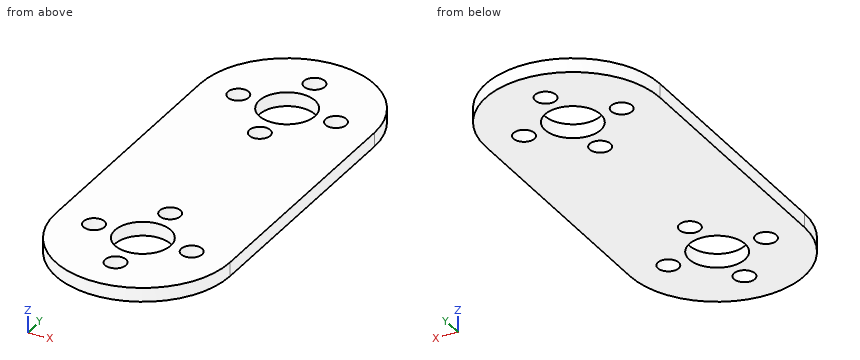
```python
from build123d import *

# Parameters (mm, degrees)
BOSS_EXTRUDE1_DEPTH     = 1
CUT_EXTRUDE1_REACH      = 53.093
SKETCH2_R               = 4
CUT_EXTRUDE2_REACH      = 53.093
SKETCH2_3_R             = 1.5
CIRPATTERN1_COUNT       = 4
MIRROR1_COPY_1_REACH    = 53.093
MIRROR1_COPY_1_SKETCH_R = 1.5
MIRROR1_COPY_2_REACH    = 53.093
MIRROR1_COPY_2_SKETCH_R = 1.5
MIRROR1_COPY_3_REACH    = 53.093
MIRROR1_COPY_3_SKETCH_R = 1.5


with BuildPart() as part:
    # Sketch1 → Boss-Extrude1 (new, symmetric)
    with BuildSketch(Plane.XY):
        with BuildLine():
            Line((-12.5, 0), (-12.5, 37))
            ThreePointArc((-12.5, 37), (0, 49.5), (12.5, 37))
            Line((12.5, 37), (12.5, 0))
            ThreePointArc((12.5, 0), (0, -12.5), (-12.5, 0))
        make_face()
    extrude(amount=BOSS_EXTRUDE1_DEPTH, both=True)

    # Sketch2 → Cut-Extrude1 (cut, up to next)
    with BuildSketch(Plane(origin=(0, 0, -1), x_dir=(-1, 0, 0), z_dir=(0, 0, -1)), mode=Mode.PRIVATE) as cut_extrude1_sk1:
        with Locations((0, 37)):
            Circle(SKETCH2_R)
    cut_extrude1_tool1 = extrude(cut_extrude1_sk1.sketch, amount=-CUT_EXTRUDE1_REACH, mode=Mode.PRIVATE) & part.part
    cut_extrude1 = cut_extrude1_tool1.solids().sort_by_distance((0, 37, -1))[0]
    add(cut_extrude1, mode=Mode.SUBTRACT)

    # Sketch2_3 → Cut-Extrude2 (cut, up to next)
    with BuildSketch(Plane(origin=(0, 0, -1), x_dir=(-1, 0, 0), z_dir=(0, 0, -1)), mode=Mode.PRIVATE) as cut_extrude2_sk1:
        with Locations((0, 44)):
            Circle(SKETCH2_3_R)
    cut_extrude2_tool1 = extrude(cut_extrude2_sk1.sketch, amount=-CUT_EXTRUDE2_REACH, mode=Mode.PRIVATE) & part.part
    cut_extrude2 = cut_extrude2_tool1.solids().sort_by_distance((0, 44, -1))[0]
    add(cut_extrude2, mode=Mode.SUBTRACT)

    # CirPattern1: Cut-Extrude2 ×4 about axis
    cirpattern1_axis = Axis((0, 37, 0), (0, 0, 1))
    for i in range(1, CIRPATTERN1_COUNT):
        add(cut_extrude2.rotate(cirpattern1_axis, i * 360 / CIRPATTERN1_COUNT), mode=Mode.SUBTRACT)

    # Mirror1: Cut-Extrude1, Cut-Extrude2 across plane
    add(cut_extrude1.mirror(Plane.ZX.offset(18.5)), mode=Mode.SUBTRACT)
    add(cut_extrude2.mirror(Plane.ZX.offset(18.5)), mode=Mode.SUBTRACT)

    # Mirror1 copy 1 sketch → Mirror1 copy 1 (cut, up to next)
    with BuildSketch(Plane(origin=(37, 0, -1), x_dir=(0, 1, 0), z_dir=(0, 0, -1)), mode=Mode.PRIVATE) as mirror1_copy_1_sk1:
        with Locations((0, -44)):
            Circle(MIRROR1_COPY_1_SKETCH_R)
    mirror1_copy_1_tool1 = extrude(mirror1_copy_1_sk1.sketch, amount=-MIRROR1_COPY_1_REACH, mode=Mode.PRIVATE) & part.part
    add(mirror1_copy_1_tool1.solids().sort_by_distance((-7, 0, -1))[0], mode=Mode.SUBTRACT)

    # Mirror1 copy 2 sketch → Mirror1 copy 2 (cut, up to next)
    with BuildSketch(Plane(origin=(0, -37, -1), x_dir=(1, 0, 0), z_dir=(0, 0, -1)), mode=Mode.PRIVATE) as mirror1_copy_2_sk1:
        with Locations((0, -44)):
            Circle(MIRROR1_COPY_2_SKETCH_R)
    mirror1_copy_2_tool1 = extrude(mirror1_copy_2_sk1.sketch, amount=-MIRROR1_COPY_2_REACH, mode=Mode.PRIVATE) & part.part
    add(mirror1_copy_2_tool1.solids().sort_by_distance((0, 7, -1))[0], mode=Mode.SUBTRACT)

    # Mirror1 copy 3 sketch → Mirror1 copy 3 (cut, up to next)
    with BuildSketch(Plane(origin=(-37, 0, -1), x_dir=(0, -1, 0), z_dir=(0, 0, -1)), mode=Mode.PRIVATE) as mirror1_copy_3_sk1:
        with Locations((0, -44)):
            Circle(MIRROR1_COPY_3_SKETCH_R)
    mirror1_copy_3_tool1 = extrude(mirror1_copy_3_sk1.sketch, amount=-MIRROR1_COPY_3_REACH, mode=Mode.PRIVATE) & part.part
    add(mirror1_copy_3_tool1.solids().sort_by_distance((7, 0, -1))[0], mode=Mode.SUBTRACT)


solid = part.part
```
Input: part model. Units: mm. Frame: model coordinates. Give positions to 0.01 mm unless a question says otherwise; leave off trailing zeros. Order: outer loops, then holes, each group sorted by start corner. A loop starts at its lowest first (then second) coordinate and runs counter-clockwise, first axis right, second up.
1. Cut plane D-D (y = -7). Return loops of the section in (x, z).
Computed:
outline: (-10.36, -1) - (-1.5, -1) - (-1.5, 1) - (-10.36, 1) - close; (1.5, -1) - (10.36, -1) - (10.36, 1) - (1.5, 1) - close
2. Pin query (flat end, axial travel): pin 1 Ø5 at (x, y) = (-7, 37) entering from +Z; pin 2 Ø1 at (x, z) = (9.5, 0) entering from +Y. Return the tip coordinate at first contact, or that it passes through.
Computed:
pin 1: stops at z = 1
pin 2: stops at y = 45.67
3. Line query: probe 1 along X at (y, z) = (30, 0.4); probe 2 along Y at (x, z) = (5.75, -0.25); probe 3 along X at (y, z) = (3.5, -0.8). Output: solid intervals per line, ascending.
Computed:
probe 1: x = -12.5 to -1.5, 1.5 to 12.5
probe 2: y = -11.1 to -0.83, 0.83 to 36.17, 37.83 to 48.1
probe 3: x = -12.5 to -1.94, 1.94 to 12.5
4. Cut plane A-A (z = 0.2). State how many separate pieces and enclosed holes the cut face has, and give its area (3 significant figures).
Computed:
separate pieces: 1
enclosed holes: 10
area: 1,260 mm2
5. Cut plane C-C (x = -7). Return loops of the section in (y, z).
Computed:
outline: (-10.36, -1) - (-1.5, -1) - (-1.5, 1) - (-10.36, 1) - close; (1.5, -1) - (35.5, -1) - (35.5, 1) - (1.5, 1) - close; (38.5, -1) - (47.36, -1) - (47.36, 1) - (38.5, 1) - close
6. Cut plane B-B (y = 7). Return loops of the section in (x, z).
Computed:
outline: (-12.5, -1) - (-1.5, -1) - (-1.5, 1) - (-12.5, 1) - close; (1.5, -1) - (12.5, -1) - (12.5, 1) - (1.5, 1) - close
